Solid Edge part; units mm, degrees
sketch "Sketch1" plane through (0, 0, 0) normal (0, 0, 1) x (1, 0, 0)
  arc A0 (-49.1, 41.5) -> (-51.1, 39.5) centre (-49.1, 39.5) ccw
  line L0 (-51.1, 39.5) -> (-51.1, -39.5)
  arc A1 (-51.1, -39.5) -> (-49.1, -41.5) centre (-49.1, -39.5) ccw
  line L1 (-49.1, -41.5) -> (49.1, -41.5)
  arc A2 (49.1, -41.5) -> (51.1, -39.5) centre (49.1, -39.5) ccw
  line L2 (51.1, -39.5) -> (51.1, 39.5)
  arc A3 (49.1, 41.5) -> (51.1, 39.5) centre (49.1, 39.5) cw
  line L3 (49.1, 41.5) -> (-49.1, 41.5)
extrude "ExtrudedProtrusion_1" add sketch "Sketch1" along normal blind 7
sketch "Sketch2" plane through (0, 0, 7) normal (0, 0, 1) x (0, -1, 0)
  arc A0 (39.5, -49.7) -> (40.1, -49.1) centre (39.5, -49.1) ccw
  line L0 (40.1, -49.1) -> (40.1, 49.1)
  arc A1 (40.1, 49.1) -> (39.5, 49.7) centre (39.5, 49.1) ccw
  line L1 (39.5, 49.7) -> (-39.5, 49.7)
  arc A2 (-39.5, 49.7) -> (-40.1, 49.1) centre (-39.5, 49.1) ccw
  line L2 (-40.1, 49.1) -> (-40.1, -49.1)
  arc A3 (-40.1, -49.1) -> (-39.5, -49.7) centre (-39.5, -49.1) ccw
  line L3 (-39.5, -49.7) -> (39.5, -49.7)
extrude "ExtrudedCutout_1" cut sketch "Sketch2" against normal blind 5.6
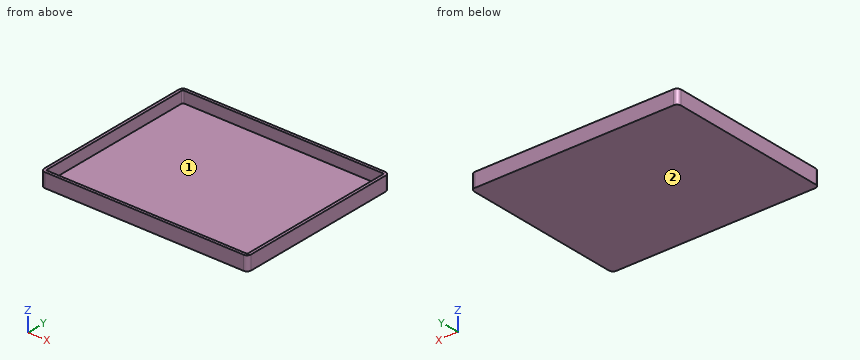
Build history of the part. All positions in model axes, mm. Face numbers are marked on the shaded views. Coordinates: 2 decimals unless noted, no trailing zeros. Write each loop counter-clockwise with the first axis right and the second up, starting at its lowest first coordinate (ties: lowest second). Pieces come first, ordered by that corner, then holes. Notation, with made-up numbers: (48, -26) -> (79, -26) arc R37 ccw to (79, 10) -> close; hole circle Ø3 at (5, 79). An arc over 180 degrees is marked (long way). Use CSV: the item, a comma, the result in double quotes. Start each with the question number.
Q1. Pull direction Y, two halves, no side cores. Call the marked faces 1 and 2: released by +Y, released by -Y, zero draft, split by the parting line, or undercut.
Q2. Cut at B-B, the plane y = -24.5. List the corners of the cut face in (x, z), then the cut area to 3 significant figures.
Q3. Cut at A-A, the plane z = 3.25. List the corners of the cut face in (x, y), then the cut area to 3 significant figures.
Q4. Flat gauge pins, fed straight in: pin 1 Ø8 at (x, y) = (16, -20) entering from -Z; pin 2 Ø6 at (x, y) = (22.5, 27) entering from +Z. Where does each tip first touch, or does it go through?
Q5. Drill centre lines: probe 1 along Y at (x, z) = (20.5, 5.75); probe 2 along X at (y, z) = (-21.5, 3); probe 3 along Z at (x, y) = (-22.5, 8.5). Where is each one in solid material? Low to high.
Q6. Cut at C-C, the plane x = -17.5. List the corners of the cut face in (y, z).
Checked values:
1,face 1,"undercut"
1,face 2,"zero draft"
2,outline,"(-51.1, 0) -> (51.1, 0) -> (51.1, 7) -> (49.7, 7) -> (49.7, 1.4) -> (-49.7, 1.4) -> (-49.7, 7) -> (-51.1, 7) -> close"
2,area,"159 mm²"
3,outline,"(-51.1, -39.5) arc R2 ccw to (-49.1, -41.5) -> (49.1, -41.5) arc R2 ccw to (51.1, -39.5) -> (51.1, 39.5) arc R2 ccw to (49.1, 41.5) -> (-49.1, 41.5) arc R2 ccw to (-51.1, 39.5) -> close; hole (-49.7, -39.5) arc R0.6 ccw to (-49.1, -40.1) -> (49.1, -40.1) arc R0.6 ccw to (49.7, -39.5) -> (49.7, 39.5) arc R0.6 ccw to (49.1, 40.1) -> (-49.1, 40.1) arc R0.6 ccw to (-49.7, 39.5) -> close"
3,area,"508 mm²"
4,pin 1,"stops at z = 0"
4,pin 2,"stops at z = 1.4"
5,probe 1,"y = -41.5 to -40.1, 40.1 to 41.5"
5,probe 2,"x = -51.1 to -49.7, 49.7 to 51.1"
5,probe 3,"z = 0 to 1.4"
6,outline,"(-41.5, 0) -> (41.5, 0) -> (41.5, 7) -> (40.1, 7) -> (40.1, 1.4) -> (-40.1, 1.4) -> (-40.1, 7) -> (-41.5, 7) -> close"
